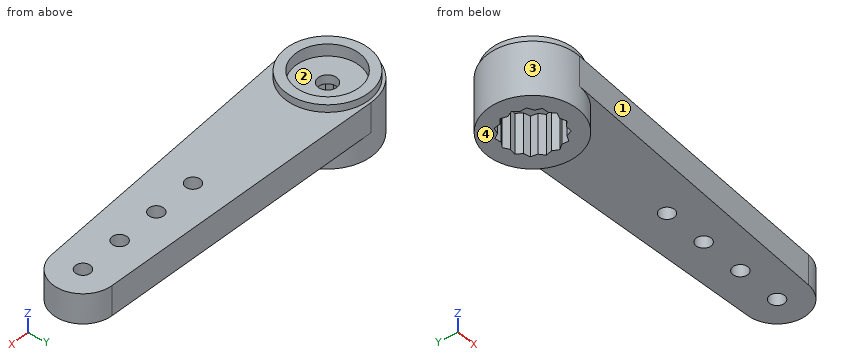
from build123d import *

# Parameters (mm, degrees)
SKETCH2_R           = 3
SKETCH2_R_2         = 2.8
BOSS_EXTRUDE1_DEPTH = 3.6
SKETCH2_3_R         = 2.8
SKETCH2_3_R_2       = 2.15
BOSS_EXTRUDE2_DEPTH = 4.1
BOSS_EXTRUDE3_START = 2.7
SKETCH2_4_R         = 2.15
SKETCH2_4_R_2       = 0.625
BOSS_EXTRUDE3_DEPTH = 0.6
SKETCH2_5_R         = 2.15
BOSS_EXTRUDE4_DEPTH = 2.7
BOSS_EXTRUDE5_START = 3.6
SKETCH2_6_R         = 0.5
BOSS_EXTRUDE5_DEPTH = 2


with BuildPart() as part:
    # Sketch2 → Boss-Extrude1 (new body)
    with BuildSketch(Plane.XY):
        Circle(SKETCH2_R)
        Circle(SKETCH2_R_2, mode=Mode.SUBTRACT)
    extrude(amount=BOSS_EXTRUDE1_DEPTH)

    # Sketch2<3> → Boss-Extrude2 (add)
    with BuildSketch(Plane.XY):
        Circle(SKETCH2_3_R)
        Circle(SKETCH2_3_R_2, mode=Mode.SUBTRACT)
    extrude(amount=BOSS_EXTRUDE2_DEPTH)

    # Sketch2<4> → Boss-Extrude3 (add)
    with BuildSketch(Plane.XY.offset(BOSS_EXTRUDE3_START)):
        Circle(SKETCH2_4_R)
        Circle(SKETCH2_4_R_2, mode=Mode.SUBTRACT)
    extrude(amount=BOSS_EXTRUDE3_DEPTH)

    # Sketch2<5> → Boss-Extrude4 (add)
    with BuildSketch(Plane.XY):
        Circle(SKETCH2_5_R)
        Polygon((-0.374241043, 1.760665681), (0, 2), (0.374241043, 1.760665681), (0.813473286, 1.827090915), (1.058013454, 1.45623059), (1.486289651, 1.338261213), (1.558845727, 0.9), (1.902113033, 0.618033989), (1.790139412, 0.188151234), (1.989043791, -0.209056927), (1.711901729, -0.55623059), (1.732050808, -1), (1.337660686, -1.204435091), (1.175570505, -1.618033989), (0.732125958, -1.644381824), (0.415823382, -1.956295201), (0, -1.8), (-0.415823382, -1.956295201), (-0.732125958, -1.644381824), (-1.175570505, -1.618033989), (-1.337660686, -1.204435091), (-1.732050808, -1), (-1.711901729, -0.55623059), (-1.989043791, -0.209056927), (-1.790139412, 0.188151234), (-1.902113033, 0.618033989), (-1.558845727, 0.9), (-1.486289651, 1.338261213), (-1.058013454, 1.45623059), (-0.813473286, 1.827090915), align=None, mode=Mode.SUBTRACT)
    extrude(amount=BOSS_EXTRUDE4_DEPTH)

    # Sketch2<6> → Boss-Extrude5 (add)
    with BuildSketch(Plane.XY.offset(BOSS_EXTRUDE5_START)):
        with BuildLine():
            Line((20.1, 1.997498436), (0.15, 2.996247653))
            ThreePointArc((0.15, 2.996247653), (3, 0), (0.15, -2.996247653))
            Line((0.15, -2.996247653), (20.1, -1.997498436))
            ThreePointArc((20.1, -1.997498436), (22, 0), (20.1, 1.997498436))
        make_face()
        with Locations((11, 0)):
            Circle(SKETCH2_6_R, mode=Mode.SUBTRACT)
        with Locations((14, 0)):
            Circle(SKETCH2_6_R, mode=Mode.SUBTRACT)
        with Locations((17, 0)):
            Circle(SKETCH2_6_R, mode=Mode.SUBTRACT)
        with Locations((20, 0)):
            Circle(SKETCH2_6_R, mode=Mode.SUBTRACT)
    extrude(amount=-BOSS_EXTRUDE5_DEPTH)


solid = part.part
Input: part model. Units: mm. Frame: model coordinates. Face numbers are marked on the shaded views. Coordinates: 2 decimals unless noted, no trailing zeros. Loops run counter-clockwise (first coordinate to the right, second up) from the corner with the lowest first, then second, coordinate; pieces in that order, holes last. Notation, with made-up numbers: (22.5, -33) -> (36.5, -33) arc R25 ccw to (36.5, 0) -> close; hole circle Ø6 at (10, 36). An arc over 180 degrees is marked (long way). One line per item, written item: value.
(1) Ray query, line 1 along Y through (x, z) = (0, 3) (3 decimals); line 2 along Z through (x, y) = (21.25, -0.75); line 3 along Y through (x, z) = (17, 2.3). Return the intervals inside material, ascending.
Answer below:
line 1: y = -3 to -0.625, 0.625 to 3
line 2: z = 1.6 to 3.6
line 3: y = -2.15 to -0.5, 0.5 to 2.15
(2) Cut plane C-C (y = 2.4). Output: boundary loops of the cut face in (x, z), then the cut area to 3 significant figures.
Answer below:
outline: (-1.8, 0) -> (1.8, 0) -> (1.8, 1.6) -> (12.06, 1.6) -> (12.06, 3.6) -> (1.44, 3.6) -> (1.44, 4.1) -> (-1.44, 4.1) -> (-1.44, 3.6) -> (-1.8, 3.6) -> close
area: 34.9 mm2
(3) Cut plane D-D (x = 11). Output: boundary loops of the cut face in (y, z).
Answer below:
outline: (-2.45, 1.6) -> (-0.5, 1.6) -> (-0.5, 3.6) -> (-2.45, 3.6) -> close; (0.5, 1.6) -> (2.45, 1.6) -> (2.45, 3.6) -> (0.5, 3.6) -> close
(4) Pin query (flat end, axial travel): pin 1 Ø2 at (x, z) = (19, 2.5) entering from -Y; pin 2 Ø1.5 at (x, y) = (13, 0.5) entering from -Z; pin 3 Ø1.8 at (x, y) = (5, -0.5) entering from +Z. Return the tip coordinate at first contact, or that it passes through.
Answer below:
pin 1: stops at y = -2.1
pin 2: stops at z = 1.6
pin 3: stops at z = 3.6
(5) Draft query along X for the marked faces 1, 2, 3 and 4. Return one class per face: pulls with the +X half, pulls with the -X half, needs draft (parallel to the pull), parting line crosses it, or undercut.
Answer below:
face 1: pulls with the +X half
face 2: undercut
face 3: parting line crosses it
face 4: needs draft
(6) Cut plane B-B (x = 14). Output: boundary loops of the cut face in (y, z).
Answer below:
outline: (-2.3, 1.6) -> (-0.5, 1.6) -> (-0.5, 3.6) -> (-2.3, 3.6) -> close; (0.5, 1.6) -> (2.3, 1.6) -> (2.3, 3.6) -> (0.5, 3.6) -> close
